```python
from build123d import *

# Parameters (mm, degrees)
CROQUIS1_W                        = 13
CROQUIS1_H                        = 12.1
SALIENTE_EXTRUIR1_DEPTH           = 11
SALIENTE_EXTRUIR2_DEPTH           = 26
CROQUIS3_R                        = 1.6
SALIENTE_EXTRUIR3_DEPTH           = 0.2
CROQUIS4_R                        = 1.5
SALIENTE_EXTRUIR4_DEPTH           = 11.5
CORTAR_EXTRUIR1_START             = -10
CORTAR_EXTRUIR1_DEPTH             = 10
CROQUIS6_W                        = 0.404320018
CROQUIS6_H                        = 2.479368964
SALIENTE_EXTRUIR5_DEPTH           = 4
CROQUIS7_W                        = 0.404320018
CROQUIS7_H                        = 2.479368964
SALIENTE_EXTRUIR6_DEPTH           = 4
CROQUIS8_W                        = 7.825868338
CROQUIS8_H                        = 23.999330497
CORTAR_EXTRUIR2_DEPTH             = 0.1
CROQUIS10_W                       = 1.15
CROQUIS10_H                       = 0.1
CROQUIS11_W                       = 1.15
CROQUIS11_H                       = 0.1
TALADRO1_D                        = 1.077216746
TALADRO1_DEPTH                    = 1.125812406
TALADRO2_D                        = 1.077216746
TALADRO2_DEPTH                    = 1.125812406
DI_METRO_DE_TALADRO_2_0_2_1_D     = 2
DI_METRO_DE_TALADRO_2_0_2_1_DEPTH = 5
DI_METRO_DE_TALADRO_2_0_2_1_TIP   = 0.600860619
CHAFL_N1_SIZE                     = 0.5
REDONDEO1_R                       = 0.5
REDONDEO2_R                       = 1


with BuildPart() as part:
    # Croquis1 → Saliente-Extruir1 (new body)
    with BuildSketch(Plane.XY):
        Rectangle(CROQUIS1_W, CROQUIS1_H)
    extrude(amount=-SALIENTE_EXTRUIR1_DEPTH)

    # Croquis2 → Saliente-Extruir2 (add)
    with BuildSketch(Plane.XY):
        with BuildLine():
            Line((-4.5, 6), (4.5, 6))
            ThreePointArc((4.5, 6), (7.5, 0), (4.5, -6))
            Line((4.5, -6), (-4.5, -6))
            ThreePointArc((-4.5, -6), (-7.5, 0), (-4.5, 6))
        make_face()
    extrude(amount=SALIENTE_EXTRUIR2_DEPTH)

    # Croquis3 → Saliente-Extruir3 (add)
    with BuildSketch(Plane(origin=(0, 0, -11), x_dir=(-1, 0, 0), z_dir=(0, 0, -1))):
        Circle(CROQUIS3_R)
    extrude(amount=SALIENTE_EXTRUIR3_DEPTH)

    # Croquis4 → Saliente-Extruir4 (add)
    with BuildSketch(Plane(origin=(0, 0, -11.2), x_dir=(-1, 0, 0), z_dir=(0, 0, -1))):
        Circle(CROQUIS4_R)
    extrude(amount=SALIENTE_EXTRUIR4_DEPTH)

    # Croquis5 → Cortar-Extruir1 (cut)
    with BuildSketch(Plane(origin=(0, 0, -22.7), x_dir=(-1, 0, 0), z_dir=(0, 0, -1)).offset(CORTAR_EXTRUIR1_START)):
        with BuildLine():
            Line((1.072168527, -1.049025571), (-1.072168527, -1.049025571))
            ThreePointArc((-1.072168527, -1.049025571), (0, -1.5), (1.072168527, -1.049025571))
        make_face()
    extrude(amount=CORTAR_EXTRUIR1_DEPTH, mode=Mode.SUBTRACT)

    # Croquis6 → Saliente-Extruir5 (add)
    with BuildSketch(Plane.XY.offset(26)):
        with Locations((-6.576347603, 0)):
            Rectangle(CROQUIS6_W, CROQUIS6_H)
    extrude(amount=SALIENTE_EXTRUIR5_DEPTH)

    # Croquis7 → Saliente-Extruir6 (add)
    with BuildSketch(Plane.XY.offset(26)):
        with Locations((6.576347603, 0)):
            Rectangle(CROQUIS7_W, CROQUIS7_H)
    extrude(amount=SALIENTE_EXTRUIR6_DEPTH)

    # Croquis8 → Cortar-Extruir2 (cut)
    with BuildSketch(Plane(origin=(0, 6, 0), x_dir=(-1, 0, 0), z_dir=(0, 1, 0))):
        with Locations((0, 12.819518154)):
            Rectangle(CROQUIS8_W, CROQUIS8_H)
    extrude(amount=-CORTAR_EXTRUIR2_DEPTH, mode=Mode.SUBTRACT)

    # Croquis9 → Revolución1 (revolve)
    with BuildSketch(Plane(origin=(0, 0, 0), x_dir=(1, 0, 0), z_dir=(0, 1, 0))):
        Polygon((4.4, -26), (0, -26), (0, -28.7), (2.375, -28.7), (2.375, -26.5), (4.4, -26.5), align=None)
    revolve(axis=Axis((0, 0, 26), (0, 0, 1)))

    # Croquis10 → Cortar-Revolución1 (revolve, cut)
    with BuildSketch(Plane(origin=(0, -4.05, 0), x_dir=(1, 0, 0), z_dir=(0, 1, 0))):
        with Locations((-3.925, 10.95)):
            Rectangle(CROQUIS10_W, CROQUIS10_H)
    revolve(axis=Axis((-4.5, -4.05, -11), (0, 0, 1)), mode=Mode.SUBTRACT)

    # Croquis11 → Cortar-Revolución2 (revolve, cut)
    with BuildSketch(Plane(origin=(0, 4.05, 0), x_dir=(1, 0, 0), z_dir=(0, 1, 0))):
        with Locations((5.075, 10.95)):
            Rectangle(CROQUIS11_W, CROQUIS11_H)
    revolve(axis=Axis((4.5, 4.05, -11), (0, 0, 1)), mode=Mode.SUBTRACT)

    # Taladro1
    with Locations(Plane(origin=(-6.374187594, 0, 0), x_dir=(0, 0, -1), z_dir=(1, 0, 0))):
        with Locations((-28.806812644, 0)):
            Hole(TALADRO1_D / 2, depth=TALADRO1_DEPTH)

    # Taladro2
    with Locations(Plane.ZY.offset(-6.374187594)):
        with Locations((28.806812644, 0)):
            Hole(TALADRO2_D / 2, depth=TALADRO2_DEPTH)

    # Diámetro de taladro Ø2.0 (2)1
    with Locations(Plane(origin=(0, 0, -11), x_dir=(-1, 0, 0), z_dir=(0, 0, -1))):
        with Locations((0, 4.375), (0, -4.375)):
            Hole(DI_METRO_DE_TALADRO_2_0_2_1_D / 2, depth=DI_METRO_DE_TALADRO_2_0_2_1_DEPTH)
            with Locations((0, 0, -(DI_METRO_DE_TALADRO_2_0_2_1_DEPTH + DI_METRO_DE_TALADRO_2_0_2_1_TIP / 2))):  # 118° drill point
                Cone(0, DI_METRO_DE_TALADRO_2_0_2_1_D / 2, DI_METRO_DE_TALADRO_2_0_2_1_TIP, mode=Mode.SUBTRACT)

    # Chaflán1
    chafl_n1_edges = [part.edges().sort_by_distance(p)[0] for p in [
        (-6.576347603, -1.239684482, 30),
        (-6.576347603, 1.239684482, 30),
        (6.576347603, 1.239684482, 30),
        (6.576347603, -1.239684482, 30),
    ]]
    chamfer(chafl_n1_edges, length=CHAFL_N1_SIZE)

    # Redondeo1
    redondeo1_edges = [part.edges().sort_by_distance(p)[0] for p in [
        (-2.375, 0, 28.7),
    ]]
    fillet(redondeo1_edges, radius=REDONDEO1_R)

    # Redondeo2
    redondeo2_edges = [part.edges().sort_by_distance(p)[0] for p in [
        (-6.5, -6.05, -5.5),
        (-6.5, 6.05, -5.5),
        (6.5, 6.05, -5.5),
        (6.5, -6.05, -5.5),
    ]]
    fillet(redondeo2_edges, radius=REDONDEO2_R)


solid = part.part
```
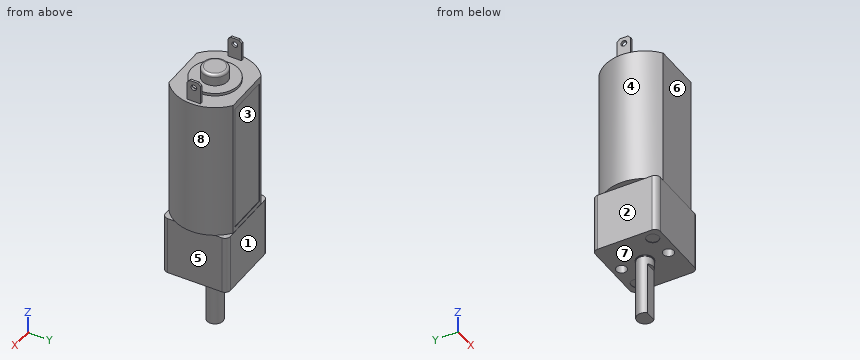
CAD build for the part. Positions are in the model's coordinates, mm. Face numbers are marked on the shaded views. A direction names the side the tool comes from. Give positions to 0.01 mm unless a question says otherwise; leave off trailing zeros. Loops run counter-clockwise (first coordinate to the right, second up) from the corner with the lowest first, then second, coordinate; pieces in that order, holes last. Notation, with made-up numbers: (54.25, 34.5) -> (97.25, 34.5) arc R19 cw to (97.25, 61.5) -> close; hole circle Ø3 at (79, 12.25). An arc over 180 degrees is marked (long way). Use a Markdown table: item, result.
1. Which spindle directions (+Z, -Z, +X, -X, +Y, -Y) get a long thin tool onto all of the face, cutting with end or side? Do the marked faces 4, 5, 6, 7 and 8. Say none if no direction does.
Check result:
| item | result |
|---|---|
| face 4 | +Z, -X |
| face 5 | -Z, +X, +Y, -Y |
| face 6 | +Z, +X, -X, -Y |
| face 7 | -Z |
| face 8 | +Z, +X |
2. Slice it at B-B (x = 5). List the corners of the cut face in (y, z), plus the area to 3 significant figures.
Check result:
| item | result |
|---|---|
| outline | (-6.05, -11) -> (3.01, -11) -> (3.01, -10.9) -> (5.09, -10.9) -> (5.09, -11) -> (6.05, -11) -> (6.05, 0) -> (5.59, 0) -> (5.59, 26) -> (-5.59, 26) -> (-5.59, 0) -> (-6.05, 0) -> close |
| area | 424 mm^2 |
3. Slice it at A-A (z = 1.5). List the corners of the cut face in (x, y), plus the area to 3 significant figures.
Check result:
| item | result |
|---|---|
| outline | (-4.5, -6) -> (4.5, -6) arc R7.5 ccw to (4.5, 6) -> (3.91, 6) -> (3.91, 5.9) -> (-3.91, 5.9) -> (-3.91, 6) -> (-4.5, 6) arc R7.5 ccw to start |
| area | 158 mm^2 |
4. Flat gauge pins, fed straight in: pin 1 (1.2 mm diameter, centred on x = 2, y = -5, fed in from +Z); pin 2 (1.5 mm diameter, centred on x = -3, z = 2.5, fed in from -Y); pin 3 (0.5 mm diameter, centred on x = -0.5, y = -1.5, fed in from -Z); pin 4 (8 mm diameter, centred on x = -6, z = -15.5, fed in from +Y). Where does each tip first touch, or does it go through?
Check result:
| item | result |
|---|---|
| pin 1 | stops at z = 26 |
| pin 2 | stops at y = -6 |
| pin 3 | stops at z = -12.7 |
| pin 4 | passes through |
5. Mould opens along X. For the marked faces 1, 2 and 3 say: pulls with the +X half, pulls with the -X half, needs draft (parallel to the pull), parting line crosses it, or undercut.
Check result:
| item | result |
|---|---|
| face 1 | needs draft |
| face 2 | pulls with the -X half |
| face 3 | undercut |
6. Wall check: L1, parallel to Y at x = 0, z = -8.4 (3 decimals); L2, parallel to X at y = -4.5, z = -9; L3, parallel to Z at x = 4, y = -3. Give the ranges that are in metal, low to high. Write a range as [from, to].
Check result:
| item | result |
|---|---|
| L1 | y = [-6.05, -5.375], [-3.375, 3.375], [5.375, 6.05] |
| L2 | x = [-6.5, -0.99], [0.99, 6.5] |
| L3 | z = [-11, 26] |
7. Slice it at C-C (y = 0). Give the number of separate pieces and of enclosed holes in the cut face, plus the area to 3 significant figures.
Check result:
| item | result |
|---|---|
| separate pieces | 3 |
| enclosed holes | 0 |
| area | 585 mm^2 |
